Autodesk Inventor part; units mm, degrees
ref_plane "Work Plane1" through (0, 9, 0) normal (0, 1, 0) x (1, 0, 0)
ref_plane "YZ Plane" through (0, 0, 0) normal (1, 0, 0) x (0, 1, 0)
ref_plane "XZ Plane" through (0, 0, 0) normal (0, 1, 0) x (-1, 0, 0)
sketch "Sketch1" plane through (0, 0, 0) normal (0, 1, 0) x (-1, 0, 0)
  line L0 (0, 0) -> (8, 0)
  line L1 (8, 0) -> (8, -26)
  line L2 (8, -26) -> (0, -26)
  line L3 (0, -26) -> (0, 0)
  dimension "d0" = 8
  dimension "d1" = 26
extrude "Extrusion1" add sketch "Sketch1" along normal blind 6
sketch "Sketch2" plane through (-8, 0, 0) normal (0, 0, 1) x (1, 0, 0)
  circle A0 centre (4, 3) radius 3
  line L0 (8, 0) -> (0, 0)
  line L1 (0, 0) -> (0, 6)
  dimension "d4" = 6
  dimension "d5" = 3
  dimension "d6" = 4
extrude "Extrusion2" add sketch "Sketch2" along normal blind 6
sketch "Sketch3" plane through (0, 0, -26) normal (0, 0, -1) x (-1, 0, 0)
  arc A0 (4, 0) -> (4, 6) centre (4, 3) ccw
  arc A1 (4, 6) -> (4, 0) centre (4, 3) ccw
  circle A2 centre (4, 3) radius 3
  point P0 (0, 0)
extrude "Extrusion3" add sketch "Sketch3" along normal blind 6
ref_plane "Work Plane1" through (0, 9, 0) normal (0, 1, 0) x (1, 0, 0)
sketch "Sketch7" plane through (0, 6, 0) normal (0, 1, 0) x (1, 0, 0)
  line L0 (-2, 13) -> (-6, 13) construction
  line L1 (-4.5266, -6) -> (-4.5266, 32)
  line L2 (-2, 14.5) -> (-6, 14.5)
  line L3 (-6, 11.5) -> (-2, 11.5)
  arc A0 (-2, 11.5) -> (-2, 14.5) centre (-2, 13) ccw
  arc A1 (-6, 14.5) -> (-6, 11.5) centre (-6, 13) ccw
  line L4 (-8, 26) -> (-8, 0)
  line L5 (-4, 0) -> (0, 0)
  point P0 (-4, 13)
  dimension "d26" = 3
  dimension "d27" = 4
  dimension "d28" = 4
  dimension "d29" = 13
sketch "Sketch8" plane through (0, 9, 0) normal (0, 1, 0) x (1, 0, 0)
  line L0 (-2, 13) -> (-6, 13) construction
  line L1 (-2, 14) -> (-6, 14)
  line L2 (-6, 12) -> (-2, 12)
  arc A0 (-2, 12) -> (-2, 14) centre (-2, 13) ccw
  arc A1 (-6, 14) -> (-6, 12) centre (-6, 13) ccw
  line L3 (-4, 13) -> (0, 13) construction
  line L4 (-8, 26) -> (-8, 0)
  line L5 (-4, 0) -> (0, 0)
  dimension "d30" = 2
  dimension "d31" = 180
  dimension "d32" = 2
  dimension "d33" = 4
  dimension "d34" = 13
loft "Loft1" add profiles "Sketch7", "Sketch8"
hole "Hole2" at (-3.899, 2.8555, -32) direction (0, 0, 1) diameter 2.5 end through all
chamfer "Chamfer1" distance 1 angle 45 1 edges at (-3.899, 1.6055, 6)
chamfer "Chamfer2" distance 1 angle 45 1 edges at (-3.899, 1.6055, -32)
fillet "Fillet1" radius 1 2 edges at (-8, 6, -13) (0, 6, -13)
properties part number "tracks_center" material "ABS Plastic"
Design review of the part built by this model. Coordinates are the model's own, in mm. A direction names the side the tool comes from. Round coordinates to 2 decimals unless told otherwise and drop trailing zeros. Loops run counter-clockwise (first coordinate to the right, second up) from the corner with the lowest first, then second, coordinate; pieces in that order, holes last. Notation, with made-up numbers: (58.25, -9.5) - (113.25, -9.5) arc R18 cw to (113.25, 6.5) - close; hole circle Ø3 at (8, 64). An arc over 180 degrees is marked (long way). One line per item, written item: value. Start each with the question number.
1) Consider section B-B on z = -20.5. Give the boundary of the cut face in (x, y).
2) To check wall thickness, follow L1, parallel to X at y = 2.75, z = -12.5; L2, parallel to Y at x = -3.75, z = -24.5; L3, parallel to Y at x = -7, z = -21. State the ranges of each line that lie inside material, in increasing order. Write a range as from..to.
3) For faces 1 (the flat face through (-0.6, 3, 0)), 2 (the flat face through (-7.4, 3, -26)), 3 (the flat face through (-0.7, 3, -26)), list the 3-axis set-ups (+Z, -Z, +X, -X, +Y, -Y) from which the entire face can be reached by the end or side of a thin tool; tool diameter is ignored.
4) Insertion check: pin 1 Ø1 at (x, z) = (-4.5, -7.5) entering from +Y; pin 2 Ø3 at (x, y) = (-3.9, 2.86) entering from +Z. Each pin has a flat end and moves straight along its axis. Give the tip position at first contact, or say it passes through.
5) Consider section C-C on z = -28. Give the boundary of the cut face in (x, y), then the cut area to 3 significant figures.
6) Consider section A-A on z = -13. Give the boundary of the cut face in (x, y).
Reported:
1. outline: (-8, 0) - (0, 0) - (0, 5) arc R1 ccw to (-1, 6) - (-7, 6) arc R1 ccw to (-8, 5) - close; hole circle Ø2.5 at (-3.9, 2.86)
2. L1: x = -8..-5.14, -2.65..0
2. L2: y = 0..1.61, 4.1..6
2. L3: y = 0..6
3. face 1: +Z, +X
3. face 2: -Z, -X
3. face 3: -Z, +X
4. pin 1: stops at y = 6
4. pin 2: stops at z = 5.25
5. outline: circle Ø6 at (-4, 3); hole circle Ø2.5 at (-3.9, 2.86)
5. area: 23.4 mm^2
6. outline: (-8, 0) - (0, 0) - (0, 5) arc R1 ccw to (-0.48, 5.85) - (-1, 9) - (-7, 9) - (-7.52, 5.85) arc R1 ccw to (-8, 5) - close; hole circle Ø2.5 at (-3.9, 2.86)
